from build123d import *

# Parameters (mm, degrees)
SKETCH1_R           = 62
SKETCH1_R_2         = 21.025
BOSS_EXTRUDE1_DEPTH = 10
SKETCH3_R           = 2.1
CUT_EXTRUDE1_DEPTH  = 89.249645892
CIRPATTERN1_COUNT   = 8
SKETCH5_R           = 4.25
CUT_EXTRUDE3_DEPTH  = 3.5
CUT_EXTRUDE2_DEPTH  = 3
CHAMFER1_SIZE       = 0.5
CHAMFER2_SIZE       = 0.5
CHAMFER3_SIZE       = 0.5
CHAMFER4_SIZE       = 0.5
CHAMFER5_SIZE       = 0.5
CHAMFER5_SIZE_2     = 0.448841824


with BuildPart() as part:
    # Sketch1 → Boss-Extrude1 (new body)
    with BuildSketch(Plane(origin=(0, 0, 0), x_dir=(1, 0, 0), z_dir=(0, 1, 0))):
        with Locations(Location((0, 0, 0), (0, 0, 270))):
            Circle(SKETCH1_R)
        with Locations(Location((0, 0, 0), (0, 0, 270))):
            Circle(SKETCH1_R_2, mode=Mode.SUBTRACT)
    extrude(amount=BOSS_EXTRUDE1_DEPTH)

    # Sketch3 → Cut-Extrude1 (cut, through all)
    with BuildSketch(Plane(origin=(0, 10, 0), x_dir=(1, 0, 0), z_dir=(0, 1, 0))):
        with Locations(Location((-56, 0, 0), (0, 0, 270))):
            Circle(SKETCH3_R)
    cut_extrude1 = extrude(amount=-CUT_EXTRUDE1_DEPTH, mode=Mode.SUBTRACT)

    # CirPattern1: Cut-Extrude1 ×8 about axis
    cirpattern1_axis = Axis((0, 0, 0), (0, 1, 0))
    for i in range(1, CIRPATTERN1_COUNT):
        add(cut_extrude1.rotate(cirpattern1_axis, i * 360 / CIRPATTERN1_COUNT), mode=Mode.SUBTRACT)

    # Sketch5 → Cut-Extrude3 (cut)
    with BuildSketch(Plane(origin=(0, 10, 0), x_dir=(1, 0, 0), z_dir=(0, 1, 0))):
        with Locations(Location((39.597979746, 39.597979746, 0), (0, 0, 270))):
            Circle(SKETCH5_R)
    extrude(amount=-CUT_EXTRUDE3_DEPTH, mode=Mode.SUBTRACT)

    # Sketch4 → Cut-Extrude2 (cut)
    with BuildSketch(Plane.XZ):
        with BuildLine():
            ThreePointArc((30.503162375, 53.977375679), (27.165020613, 55.732052314), (23.72637336, 57.280530787))
            ThreePointArc((23.72637336, 57.280530787), (20.1999424, 58.617082212), (16.59877541, 59.736761336))
            Line((16.59877541, 59.736761336), (4.528309489, 30.596078804))
            Line((4.528309489, 30.596078804), (18.432696453, 24.836693147))
            Line((18.432696453, 24.836693147), (30.503162375, 53.977375679))
        make_face()
    extrude(amount=-CUT_EXTRUDE2_DEPTH, mode=Mode.SUBTRACT)

    # Chamfer1
    chamfer1_edges = [part.edges().sort_by_distance(p)[0] for p in [
        (39.597979746, 10, -43.847979746),
        (41.082903987, 6.5, -38.113055506),
    ]]
    chamfer(chamfer1_edges, length=CHAMFER1_SIZE)

    # CirPattern2: read off the stored shape, not the designer's step
    # CirPattern2 outline → CirPattern2 (revolve, cut)
    with BuildSketch(Plane.XY.offset(56)):
        Polygon((2.1, 10), (2.1, 6.5), (4.25, 6.5), (4.25, 9.5), (4.75, 10), align=None)
    revolve(axis=Axis((0, 0, 56), (0, 1, 0)), mode=Mode.SUBTRACT)

    # CirPattern2 2 outline → CirPattern2 2 (revolve, cut)
    with BuildSketch(Plane(origin=(39.597979746, 0, 39.597979746), x_dir=(1, 0, 0), z_dir=(0, 0, 1))):
        Polygon((2.1, 10), (2.1, 6.5), (4.25, 6.5), (4.25, 9.5), (4.75, 10), align=None)
    revolve(axis=Axis((39.597979746, 0, 39.597979746), (0, 1, 0)), mode=Mode.SUBTRACT)

    # CirPattern2 3 outline → CirPattern2 3 (revolve, cut)
    with BuildSketch(Plane(origin=(56, 0, 0), x_dir=(1, 0, 0), z_dir=(0, 0, 1))):
        Polygon((2.1, 10), (2.1, 6.5), (4.25, 6.5), (4.25, 9.5), (4.75, 10), align=None)
    revolve(axis=Axis((56, 0, 0), (0, 1, 0)), mode=Mode.SUBTRACT)

    # CirPattern2 4 outline → CirPattern2 4 (revolve, cut)
    with BuildSketch(Plane.XY.offset(-56)):
        Polygon((2.1, 10), (2.1, 6.5), (4.25, 6.5), (4.25, 9.5), (4.75, 10), align=None)
    revolve(axis=Axis((0, 0, -56), (0, 1, 0)), mode=Mode.SUBTRACT)

    # CirPattern2 5 outline → CirPattern2 5 (revolve, cut)
    with BuildSketch(Plane(origin=(-39.597979746, 0, -39.597979746), x_dir=(1, 0, 0), z_dir=(0, 0, 1))):
        Polygon((2.1, 10), (2.1, 6.5), (4.25, 6.5), (4.25, 9.5), (4.75, 10), align=None)
    revolve(axis=Axis((-39.597979746, 0, -39.597979746), (0, 1, 0)), mode=Mode.SUBTRACT)

    # CirPattern2 6 outline → CirPattern2 6 (revolve, cut)
    with BuildSketch(Plane(origin=(-39.597979746, 0, 39.597979746), x_dir=(1, 0, 0), z_dir=(0, 0, 1))):
        Polygon((2.1, 10), (2.1, 6.5), (4.25, 6.5), (4.25, 9.5), (4.75, 10), align=None)
    revolve(axis=Axis((-39.597979746, 0, 39.597979746), (0, 1, 0)), mode=Mode.SUBTRACT)

    # CirPattern2 7 outline → CirPattern2 7 (revolve, cut)
    with BuildSketch(Plane(origin=(-56, 0, 0), x_dir=(1, 0, 0), z_dir=(0, 0, 1))):
        Polygon((2.1, 10), (2.1, 6.5), (4.25, 6.5), (4.25, 9.5), (4.75, 10), align=None)
    revolve(axis=Axis((-56, 0, 0), (0, 1, 0)), mode=Mode.SUBTRACT)

    # Chamfer2
    chamfer2_edges = [part.edges().sort_by_distance(p)[0] for p in [
        (38.113055505, 6.5, 41.082903986),
        (56, 6.5, 2.1),
        (2.1, 6.5, -56),
        (-38.113055505, 6.5, -41.082903986),
        (-56, 6.5, -2.1),
        (-41.082903986, 6.5, 38.113055505),
        (-2.1, 6.5, 56),
    ]]
    chamfer(chamfer2_edges, length=CHAMFER2_SIZE)

    # Chamfer3
    chamfer3_edges = [part.edges().sort_by_distance(p)[0] for p in [
        (0, 0, -21.025),
        (0, 10, -21.025),
    ]]
    chamfer(chamfer3_edges, length=CHAMFER3_SIZE)

    # Chamfer4
    chamfer4_edges = [part.edges().sort_by_distance(p)[0] for p in [
        (24.467929414, 0, 39.407034413),
        (10.56354245, 0, 45.16642007),
        (11.480502971, 0, 27.716385975),
    ]]
    chamfer(chamfer4_edges, length=CHAMFER4_SIZE)

    # Chamfer5
    # the kernel refuses this chamfer: 0.5, 0.448841824 mm, written as the material it takes off along each edge
    with BuildSketch(Plane(origin=(30.503162375, -0.785841494, 53.977375679), x_dir=(0.868821324088061, 0, -0.49512574848200785), z_dir=(0, 1, 0))) as chamfer5_piece_1:
        with BuildLine():
            Line((0.447581222, 0), (CHAMFER5_SIZE * 0.124953018626, CHAMFER5_SIZE * 0.992162659616))
            Line((CHAMFER5_SIZE * 0.124953018626, CHAMFER5_SIZE * 0.992162659616), (0, 0))
            ThreePointArc((0, 0), (0.229921968, -0.000403587), (0.447581222, 0))
        make_face()
    extrude(amount=3.785841494, mode=Mode.SUBTRACT)
    with BuildSketch(Plane(origin=(0, 3, 0), x_dir=(0.5099353263138355, 0, 0.8602127428591152), z_dir=(0.8602127428591152, 0, -0.5099353263138355))) as chamfer5_piece_2_section:
        Polygon((62, -CHAMFER5_SIZE), (62 - CHAMFER5_SIZE, 0), (62, 0), align=None)
    chamfer5_piece_2 = revolve(axis=Axis((0, 3, 0), (0, -1, 0)), revolution_arc=16.319043914, mode=Mode.PRIVATE)
    chamfer5_piece_2 = split(chamfer5_piece_2, bisect_by=Plane(origin=(-6.952193482, 3, 2.879692829), z_dir=(0.9238795325112891, 0, -0.3826834323650844)), keep=Keep.TOP, mode=Mode.PRIVATE)
    chamfer5_piece_2 = split(chamfer5_piece_2, bisect_by=Plane(origin=(6.952193482, 3, -2.879692829), z_dir=(-0.923879532511289, 0, 0.38268343236508445)), keep=Keep.TOP, mode=Mode.PRIVATE)
    add(chamfer5_piece_2, mode=Mode.SUBTRACT)
    with BuildSketch(Plane(origin=(16.59877541, -0.780714965, 59.736761336), x_dir=(-0.9645635955346866, 0, 0.26385046933670087), z_dir=(0, 1, 0))) as chamfer5_piece_3:
        with BuildLine():
            Line((0.498003952, 0), (CHAMFER5_SIZE_2 * 0.125356459071, -CHAMFER5_SIZE_2 * 0.992111765865))
            Line((CHAMFER5_SIZE_2 * 0.125356459071, -CHAMFER5_SIZE_2 * 0.992111765865), (0, 0))
            ThreePointArc((0, 0), (0.256043839, 0.000499618), (0.498003952, 0))
        make_face()
    extrude(amount=3.780714965, mode=Mode.SUBTRACT)
    with BuildSketch(Plane(origin=(0, 3, 0), x_dir=(0.5099353263138355, 0, 0.8602127428591152), z_dir=(0.8602127428591152, 0, -0.5099353263138355))) as chamfer5_piece_4a_section:
        Polygon((62, -CHAMFER5_SIZE), (62 - CHAMFER5_SIZE, 0), (62, 0), align=None)
    chamfer5_piece_4a = revolve(axis=Axis((0, 3, 0), (0, -1, 0)), revolution_arc=16.319043914, mode=Mode.PRIVATE)
    chamfer5_piece_4a = split(chamfer5_piece_4a, bisect_by=Plane(origin=(6.952193482, 3, -2.879692829), z_dir=(0.923879532511289, 0, -0.38268343236508445)), keep=Keep.TOP, mode=Mode.PRIVATE)
    with BuildSketch(Plane(origin=(30.503162375, -0.785841494, 53.977375679), x_dir=(0.868821324088061, 0, -0.49512574848200785), z_dir=(0, 1, 0))) as chamfer5_piece_4b_section:
        with BuildLine():
            Line((0.447581222, 0), (CHAMFER5_SIZE * 0.124953018626, CHAMFER5_SIZE * 0.992162659616))
            Line((CHAMFER5_SIZE * 0.124953018626, CHAMFER5_SIZE * 0.992162659616), (0, 0))
            ThreePointArc((0, 0), (0.229921968, -0.000403587), (0.447581222, 0))
        make_face()
    chamfer5_piece_4b = extrude(amount=5.071682988, mode=Mode.PRIVATE)
    chamfer5_piece_4b = split(chamfer5_piece_4b, bisect_by=Plane(origin=(30.503162375, 3, 53.977375679), z_dir=(0, 1, 0)), keep=Keep.TOP, mode=Mode.PRIVATE)
    chamfer5_piece_4 = chamfer5_piece_4a & chamfer5_piece_4b
    add(chamfer5_piece_4, mode=Mode.SUBTRACT)
    with BuildSketch(Plane(origin=(16.59877541, -0.780714965, 59.736761336), x_dir=(-0.9645635955346866, 0, 0.26385046933670087), z_dir=(0, 1, 0))) as chamfer5_piece_5a_section:
        with BuildLine():
            Line((0.498003952, 0), (CHAMFER5_SIZE_2 * 0.125356459071, -CHAMFER5_SIZE_2 * 0.992111765865))
            Line((CHAMFER5_SIZE_2 * 0.125356459071, -CHAMFER5_SIZE_2 * 0.992111765865), (0, 0))
            ThreePointArc((0, 0), (0.256043839, 0.000499618), (0.498003952, 0))
        make_face()
    chamfer5_piece_5a = extrude(amount=5.06142993, mode=Mode.PRIVATE)
    chamfer5_piece_5a = split(chamfer5_piece_5a, bisect_by=Plane(origin=(16.59877541, 3, 59.736761336), z_dir=(0, 1, 0)), keep=Keep.TOP, mode=Mode.PRIVATE)
    with BuildSketch(Plane(origin=(0, 3, 0), x_dir=(0.5099353263138355, 0, 0.8602127428591152), z_dir=(0.8602127428591152, 0, -0.5099353263138355))) as chamfer5_piece_5b_section:
        Polygon((62, -CHAMFER5_SIZE), (62 - CHAMFER5_SIZE, 0), (62, 0), align=None)
    chamfer5_piece_5b = revolve(axis=Axis((0, 3, 0), (0, -1, 0)), revolution_arc=16.319043914, mode=Mode.PRIVATE)
    chamfer5_piece_5b = split(chamfer5_piece_5b, bisect_by=Plane(origin=(-6.952193482, 3, 2.879692829), z_dir=(-0.9238795325112891, 0, 0.3826834323650844)), keep=Keep.TOP, mode=Mode.PRIVATE)
    chamfer5_piece_5 = chamfer5_piece_5a & chamfer5_piece_5b
    add(chamfer5_piece_5, mode=Mode.SUBTRACT)


solid = part.part
Design review of the part built by this model. Coordinates are the model's own, in mm. A direction names the side the tool comes from. Give positions to 0.01 mm unless a question says otherwise; leave off trailing zeros. Loops run counter-clockwise (first coordinate to the right, second up) from the corner with the lowest first, then second, coordinate; pieces in that order, holes last. Notation, with made-up numbers: M 89,45 L 123,45 A12 ccw 123,50 Z; hole C 71,24.25 d11. An arc over 180 degrees is marked long. Answer as a JSON object with one key per item and string values.
Item 1: For P1, Ø5, axis at x = 40.5, y = 7, coming from the +Z side; P2, Ø4, axis at y = 1, z = 38.5, coming from the +X side; P3, Ø4, axis at x = 42, y = 6, coming from the -Z side, all flat-tipped, find the tip position at first contact; note any pin that passes through.
Output values:
{"P1": "stops at z = 48.99", "P2": "stops at x = 50.12", "P3": "stops at z = -47.37"}
Item 2: We need section C-C (y = 8). Count the separate pieces of the cut face and the enclosed holes in it, and give its area (3 significant figures).
Output values:
{"separate pieces": "1", "enclosed holes": "9", "area": "10,200 mm2"}
Item 3: Wall thickness on line 1 along X through (y, z) = (7.9, 0) (3 decimals); line 2 along Z through (x, y) = (39, 7); line 3 along Z through (x, y) = (-56, 8.15): over which ranges is each line inside the solid? List them lowest first.
Output values:
{"line 1": "x = -62 to -60.25, -51.75 to -21.025, 21.025 to 51.75, 60.25 to 62", "line 2": "z = -48.2 to -43.81, -35.39 to 35.39, 43.81 to 48.2", "line 3": "z = -26.61 to -4.25, 4.25 to 26.61"}
Item 4: We need section B-B (z = -56). State the section outline as (x, y) points.
Output values:
{"outline": "M -26.61,0 L -2.1,0 L -2.1,6 L -2.6,6.5 L -4.25,6.5 L -4.25,9.5 L -4.75,10 L -26.61,10 Z; M 2.1,0 L 26.61,0 L 26.61,10 L 4.75,10 L 4.25,9.5 L 4.25,6.5 L 2.6,6.5 L 2.1,6 Z"}
Item 5: We need section A-A (x = 56). State the section outline as (y, z) points, and give its area (3 significant figures).
Output values:
{"outline": "M 0,-26.61 L 10,-26.61 L 10,-4.75 L 9.5,-4.25 L 6.5,-4.25 L 6.5,-2.6 L 6,-2.1 L 0,-2.1 Z; M 0,2.1 L 6,2.1 L 6.5,2.6 L 6.5,4.25 L 9.5,4.25 L 10,4.75 L 10,26.61 L 0,26.61 Z", "area": "475 mm2"}
Item 6: Mouldability with a two-part tool opening along Z and no side actions: class faces 1 (the face through (58.05, 3.04, 0.46)), 2 (the face through (-27, 0, -1)), 3 (the face through (2.73, 4.93, -61.94)) as pulls with the +Z half, pulls with the -Z half, needs draft (parallel to the pull), parting line crosses it, or undercut.
Output values:
{"face 1": "undercut", "face 2": "needs draft", "face 3": "parting line crosses it"}
Item 7: We need section D-D (z = 28). State the section outline as (x, y) points, and give its area (3 significant figures).
Output values:
{"outline": "M -55.32,0 L 9.49,0 L 10.8,0.5 L 10.8,3 L 19.74,3 L 19.74,0.5 L 20.28,0 L 55.32,0 L 55.32,10 L -55.32,10 Z", "area": "1,080 mm2"}
Item 8: Machinability: for faces 4 (the face through (-0.92, 8.02, -51.85)), 5 (the face through (11.38, 1.73, 27.76)), 6 (the face through (-37.5, 3, -39.7)), which of the approach directions +Z, -Z, +X, -X, +Y, -Y give a long, thin tool a straight path to every point of the face, cutting with its end or side? Answer none if there is none.
Output values:
{"face 4": "+Y", "face 5": "-Y", "face 6": "+Y, -Y"}
